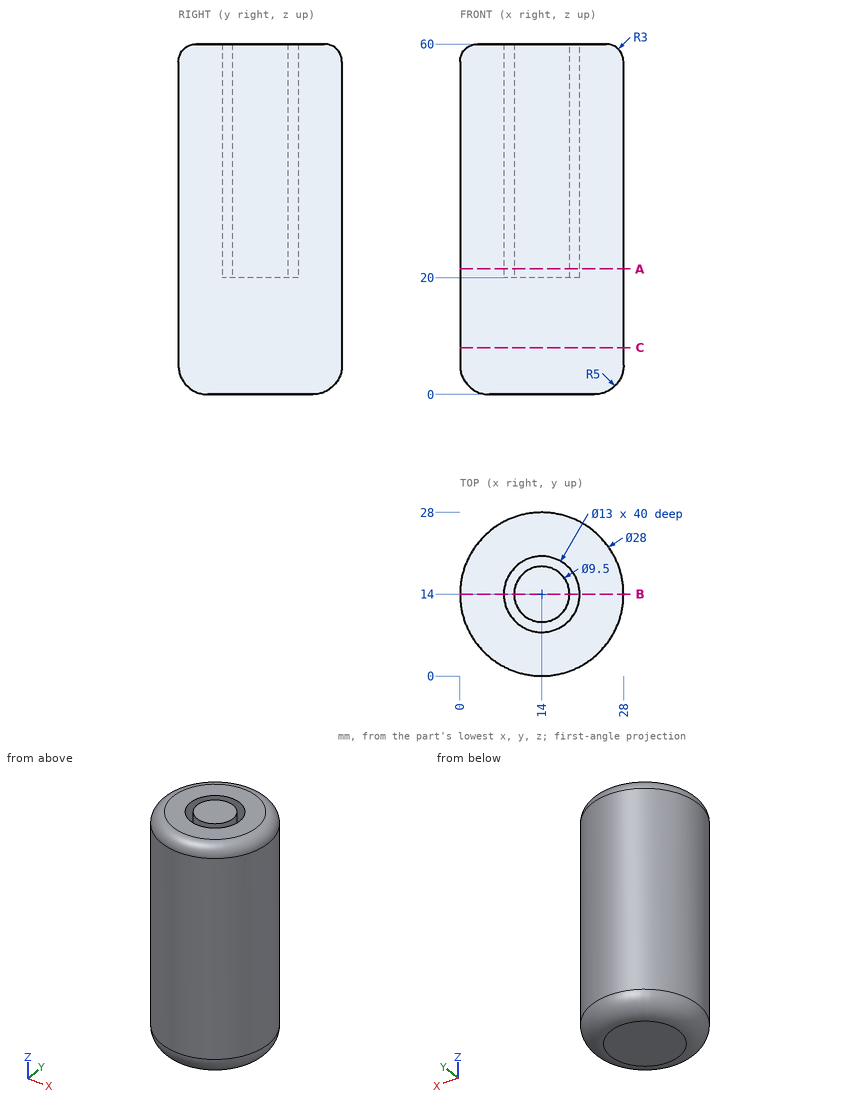
The drawing under review shows one solid part. Ordinate dimensions are in mm from its lowest x, y, z. Coordinates: 2 decimals unless noted, no trailing zeros. Write each loop counter-clockwise with the first axis right and the second up, starting at its lowest first coordinate (ties: lowest second). Pieces come first, ordered by that corner, then holes. Notation, with made-up numbers: (4, 57) - (23, 57) arc R22 ccw to (23, 86) - close; hole circle Ø3 at (-12.5, -33). An arc over 180 degrees is marked (long way). Answer in a Markdown table with one row per item. Add a question column.
Q1. We need section C-C, the plane z = 8. State the section outline as (x, y) points.
Q2. For probe 1 along Y at (x, z) = (14, 32.5); probe 2 along Y at (x, z) = (15.75, 50); probe 3 along X at (y, z) = (12.5, 56.5), list the stretches that pass through material, from the lowest coordinate up.
Q3. We need section A-A, the plane z = 21.5. State the section outline as (x, y) points.
Q4. For P1, Ø3, axis at y = 24, z = 18.5, coming from the -X side; P2, Ø2, axis at y = 7, z = 34, coming from the +X side; P3, Ø5, axis at y = 19, z = 29.5, coming from the -X side (3 decimals), all flat-tipped, find the tip position at first contact; note any pin that passes through.
Q5. We need section B-B, the plane y = 14. State the section outline as (x, z) points.
Answer list:
| question | item | result |
|---|---|---|
| 1 | outline | circle Ø28 at (14, 14) |
| 2 | probe 1 | y = 0 to 7.5, 9.25 to 18.75, 20.5 to 28 |
| 2 | probe 2 | y = 0.11 to 7.74, 9.58 to 18.42, 20.26 to 27.89 |
| 2 | probe 3 | x = 0.08 to 7.68, 9.49 to 18.51, 20.32 to 27.92 |
| 3 | outline | circle Ø28 at (14, 14); circle Ø9.5 at (14, 14); hole circle Ø13 at (14, 14) |
| 4 | P1 | stops at x = 2.88 |
| 4 | P2 | stops at x = 26.65 |
| 4 | P3 | stops at x = 0.225 |
| 5 | outline | (0, 5) arc R5 ccw to (5, 0) - (23, 0) arc R5 ccw to (28, 5) - (28, 57) arc R3 ccw to (25, 60) - (20.5, 60) - (20.5, 20) - (18.75, 20) - (18.75, 60) - (9.25, 60) - (9.25, 20) - (7.5, 20) - (7.5, 60) - (3, 60) arc R3 ccw to (0, 57) - close |
